Input: part model. Units: mm. Frame: model coordinates. Face numbers are marked on the shaded views. A direction names the side the tool comes from. Coordinates: 2 decimals unless noted, no trailing zeros. Write each loop counter-clockwise with the first axis right and the second up, starting at its lowest first coordinate (ties: lowest second). Pieces come first, ordered by that corner, then holes. Notation, with made-up numbers: M -22.75,47.5 L -9.75,47.5 A14 cw -9.75,69.5 Z; hole C 49,-5.75 d3. An arc over 180 degrees is marked long. Write each question's results on one line, items separated by ' | '. Start each with the question number.
1. Section query A-A, the plane z = 8.75. Output: boundary loops of the cut face in (x, y).
2. Pull-direction query (Y, two-part tool) for the marked faces 1, 2, 3 and 4; classes: +Y half, -Y half, draft (parallel to the pull), parting line (faces both ways), or undercut.
3. Section query D-D, the plane x = 35. Output: boundary loops of the cut face in (y, z).
4. Section query C-C, the plane z = 22. Output: boundary loops of the cut face in (x, y), and give its area (3 significant figures).
5. Section query B-B, the plane x = 0. Output: boundary loops of the cut face in (y, z), and give its area (3 significant figures).
6. Set-up query: the marked faces 5 and 6. Return all of +Z, -Z, +X, -X, +Y, -Y with unobstructed straight access to the full face (end or side cutting, diameter ignored); none if empty.
7. Ray query, probe 1 along X at (y, z) = (-0.5, 20.5); probe 2 along Y at (x, z) = (0, 14); probe 3 along X at (y, z) = (-3.75, 8.25). Return the intervals inside material, ascending.
8. First-contact query: pin 1 (12 mm diameter, centred on x = 24.5, y = 6, fed in from -Z); pin 2 (4 mm diameter, centred on x = 5.5, z = 20, fed in from +Y); pin 3 (8 mm diameter, centred on x = -35, y = 0, fed in from +Z); pin 4 (9 mm diameter, centred on x = -25.5, y = -7, fed in from +Z). Flat tips, straight axial feed; report the tip coordinate or a pass-through.
```python
from build123d import *

# Parameters (mm, degrees)
F1_DEPTH  = 10
F2_R      = 15
F3_DEPTH  = 14
F4_R      = 4.5
F5_DEPTH  = 5
F7_R      = 3
F8_DEPTH  = 27.2
F10_R     = 12
F11_DEPTH = 5
F13_R     = 10
F14_DEPTH = 25
F16_R     = 1


with BuildPart() as f1:
    # F0 (on Top) → F1 (new body)
    with BuildSketch(Plane.XY):
        with BuildLine():
            ThreePointArc((3.428571, -14.602907), (11.756457, -9.315885), (15, 0))
            ThreePointArc((15, 0), (11.756457, 9.315885), (3.428571, 14.602907))
            ThreePointArc((3.428571, 14.602907), (0, 15), (-3.428571, 14.602907))
            ThreePointArc((-3.428571, 14.602907), (-15, 0), (-3.428571, -14.602907))
            ThreePointArc((-3.428571, -14.602907), (0, -15), (3.428571, -14.602907))
        make_face()
        with BuildLine():
            ThreePointArc((3.428571, 14.602907), (11.756457, 9.315885), (15, 0))
            ThreePointArc((15, 0), (11.756457, -9.315885), (3.428571, -14.602907))
            Line((3.428571, -14.602907), (36.6, -6.81469))
            ThreePointArc((36.6, -6.81469), (28, 0), (36.6, 6.81469))
            Line((36.6, 6.81469), (3.428571, 14.602907))
        make_face()
        with BuildLine():
            ThreePointArc((-3.428571, -14.602907), (-15, 0), (-3.428571, 14.602907))
            Line((-3.428571, 14.602907), (-36.6, 6.81469))
            ThreePointArc((-36.6, 6.81469), (-30.652587, 5.486347), (-28, 0))
            ThreePointArc((-28, 0), (-30.652587, -5.486347), (-36.6, -6.81469))
            Line((-36.6, -6.81469), (-3.428571, -14.602907))
        make_face()
        with BuildLine():
            ThreePointArc((42, 0), (40.486347, 4.347413), (36.6, 6.81469))
            ThreePointArc((36.6, 6.81469), (28, 0), (36.6, -6.81469))
            ThreePointArc((36.6, -6.81469), (40.486347, -4.347413), (42, 0))
        make_face()
        with BuildLine():
            ThreePointArc((-28, 0), (-30.652587, 5.486347), (-36.6, 6.81469))
            ThreePointArc((-36.6, 6.81469), (-42, 0), (-36.6, -6.81469))
            ThreePointArc((-36.6, -6.81469), (-30.652587, -5.486347), (-28, 0))
        make_face()
    extrude(amount=F1_DEPTH)

    # F2 (on face) → F3 (join)
    with BuildSketch(Plane.XY.offset(10)):
        Circle(F2_R)
    extrude(amount=F3_DEPTH)


with BuildPart() as f5:
    # F4 (on face) → F5 (new body)
    with BuildSketch(Plane.XY.offset(10)):
        with Locations((-35, 0)):
            Circle(F4_R)
        with Locations((35, 0)):
            Circle(F4_R)
    extrude(amount=-F5_DEPTH)


with BuildPart() as f1_1:
    add(f1.part)

    # F6: cut F5
    add(f5.part, mode=Mode.SUBTRACT)


with BuildPart() as f8:
    # F7 (on face) → F8 (new body)
    with BuildSketch(Plane.XY.offset(5)):
        with Locations((-35, 0)):
            Circle(F7_R)
        with Locations((35, 0)):
            Circle(F7_R)
    extrude(amount=-F8_DEPTH)


with BuildPart() as f1_2:
    add(f1_1.part)

    # F9: cut F8
    add(f8.part, mode=Mode.SUBTRACT)


with BuildPart() as f11:
    # F10 (on face) → F11 (new body)
    with BuildSketch(Plane.XY.offset(24)):
        Circle(F10_R)
    extrude(amount=-F11_DEPTH)


with BuildPart() as f1_3:
    add(f1_2.part)

    # F12: cut F11
    add(f11.part, mode=Mode.SUBTRACT)


with BuildPart() as f14:
    # F13 (on face) → F14 (new body)
    with BuildSketch(Plane.XY.offset(19)):
        Circle(F13_R)
    extrude(amount=-F14_DEPTH)


with BuildPart() as f1_4:
    add(f1_3.part)

    # F15: cut F14
    add(f14.part, mode=Mode.SUBTRACT)

    # F16
    f16_edges = [f1_4.edges().sort_by_distance(p)[0] for p in [
        (-15, 0, 24),
    ]]
    fillet(f16_edges, radius=F16_R)


solid = f1_4.part
```
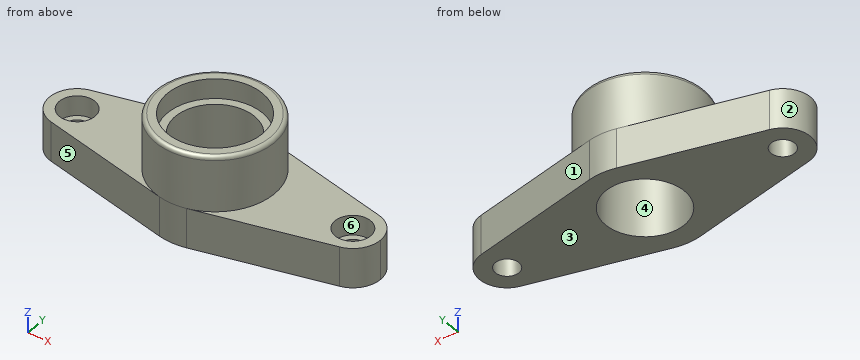
Answer:
1) outline: M -36.6,-6.81 L -3.43,-14.6 A15 ccw 3.43,-14.6 L 36.6,-6.81 A7 ccw 42,0 A7 ccw 36.6,6.81 L 3.43,14.6 A15 ccw -3.43,14.6 L -36.6,6.81 A7 ccw Z; hole C -35,0 d9; hole C 0,0 d20; hole C 35,0 d9
2) face 1: +Y half | face 2: parting line | face 3: draft | face 4: undercut
3) outline: M -7.19,0 L -3,0 L -3,5 L -4.5,5 L -4.5,10 L -7.19,10 Z; M 3,0 L 7.19,0 L 7.19,10 L 4.5,10 L 4.5,5 L 3,5 Z
4) outline: C 0,0 d30; hole C 0,0 d24 | area: 254 mm^2
5) outline: M -15,0 L -10,0 L -10,19 L -12,19 L -12,24 L -14,24 A1 ccw -15,23 Z; M 10,0 L 15,0 L 15,23 A1 ccw 14,24 L 12,24 L 12,19 L 10,19 Z | area: 220 mm^2
6) face 5: +Z, -Z, -X, -Y | face 6: +Z
7) probe 1: -14.99 to -11.99, 11.99 to 14.99 | probe 2: -15 to -10, 10 to 15 | probe 3: -40.91 to -37.49, -32.51 to -9.27, 9.27 to 32.51, 37.49 to 40.91
8) pin 1: z = 0 | pin 2: y = 14.59 | pin 3: z = 5 | pin 4: z = 10
